from build123d import *

# Parameters (mm, degrees)
SKETCH1_R                      = 3.175
BOSS_EXTRUDE1_DEPTH            = 6.35
M2_CLEARANCE_HOLE1_D           = 2.4
M2_CLEARANCE_HOLE1_CSINK_D     = 2.45
M2_CLEARANCE_HOLE1_CSINK_ANGLE = 90


with BuildPart() as part:
    # Sketch1 → Boss-Extrude1 (new body)
    with BuildSketch(Plane.XY):
        Polygon((25.4, -6.35), (25.4, -7.9375), (-25.4, -7.9375), (-25.4, -6.35), (-19.05, -6.35), (-19.05, 6.35), (-25.4, 6.35), (-25.4, 7.9375), (25.4, 7.9375), (25.4, 6.35), (19.05, 6.35), (19.05, -6.35), align=None)
        Circle(SKETCH1_R, mode=Mode.SUBTRACT)
    extrude(amount=BOSS_EXTRUDE1_DEPTH)

    # Sketch4 → Tap Drill for #6-32 Tap1 (revolve, cut)
    with BuildSketch(Plane(origin=(19.05, 0, 3.175), x_dir=(0, 0, -1), z_dir=(0, 1, 0))):
        Polygon((0, 0), (0, 7.16269403), (1.35255, 6.35), (1.35255, 0), align=None)
    tap_drill_for_6_32_tap1 = revolve(axis=Axis((25.4, 0, 3.175), (-1, 0, 0)), mode=Mode.SUBTRACT)

    # M2 Clearance Hole1 (through all)
    with Locations(Plane(origin=(0, 0, 0), x_dir=(-1, 0, 0), z_dir=(0, 0, -1))):
        with Locations((-5.5, 0), (5.5, 0)):
            CounterSinkHole(M2_CLEARANCE_HOLE1_D / 2, M2_CLEARANCE_HOLE1_CSINK_D / 2, counter_sink_angle=M2_CLEARANCE_HOLE1_CSINK_ANGLE)

    # Mirror1: Tap Drill for #6-32 Tap1 across plane
    add(tap_drill_for_6_32_tap1.mirror(Plane.ZY), mode=Mode.SUBTRACT)


solid = part.part
Can you work these out from the model? Positions are in its coordinate system, mm. A direction names the side the tool comes from. Coordinates: 2 decimals unless noted, no trailing zeros. Order: outer loops, then holes, each group sorted by start corner. A loop starts at its lowest first (then second) coordinate and runs counter-clockwise, first axis right, second up. Notation, with made-up numbers: M -26,12 L -20,12 A15 ccw -20,34 Z; hole C 65.25,-5 d1. An arc over 180 degrees is marked long. Write item = value, one per line.
(1) Suppose I cut it at B-B on z = 1. State how many separate pieces and enclosed holes the cut face has, plus the area to 3 significant figures.
Results are:
separate_pieces = 1
enclosed_holes = 3
area = 604 mm2
(2) If we mould it in two halves opening along X, with no side actions, what happens to faces 1 (the face through (0, -7.938, 3)), 2 (the face through (19.05, 2, 3)), 3 (the face through (-6.7, 0.05, 3.23))? For each: pulls with the +X half, pulls with the -X half, needs draft (parallel to the pull), parting line crosses it, or undercut.
Results are:
face_1 = needs draft
face_2 = pulls with the +X half
face_3 = undercut
(3) For faces 4 (the face through (-19.05, -2, 3)), 5 (the face through (-12.028, 0.09, 2.958)), 6 (the face through (15.919, -0.059, 4.526)), 7 (the face through (22, 6.35, 3)), 8 (the face through (0.4, -3.4, 6.35)), which set-ups out of +Z, -Z, +X, -X, +Y, -Y let a thin tool reach every point of the face, with its end or its side?
Results are:
face_4 = +Z, -Z, -X
face_5 = -X
face_6 = +X
face_7 = +Z, -Z, +X
face_8 = +Z, +X, -X, +Y, -Y
(4) Suppose I cut it at C-C on y = -2. Please give me the cut outline in (x, z), plus the area to 3 significant figures.
Results are:
outline = M -19.05,0 L -2.47,0 L -2.47,6.35 L -19.05,6.35 Z; M 2.47,0 L 19.05,0 L 19.05,6.35 L 2.47,6.35 Z
area = 211 mm2
(5) For pin 1 Ø3 at (y, z) = (3, 1.5) entering from -X; pin 2 Ø3 at (y, z) = (0, 3.175) entering from +X; pin 3 Ø1.6 at (y, z) = (0, 3.175) entering from +X; pin 4 Ø5 at (x, y) = (-7.5, 1) entering from -Z, each with a flat end and sliding along its axis, tell me the tip position at first contact or that it passes through.
Results are:
pin_1 = -19.05
pin_2 = 19.05
pin_3 = 12.37
pin_4 = 0
(6) I need wall thicknesses on line 1 along Y through (x, z) = (0, 2.25) (1 decimal); line 2 along Z through (x, y) = (-15.5, 0); line 3 along Y through (x, z) = (-5.5, 2.5). Which ranges of each line are inside material? Lowest first, please. Write a range as [from, to].
Results are:
line_1 = [-7.9, -3.2], [3.2, 7.9]
line_2 = [0, 1.82], [4.53, 6.35]
line_3 = [-7.94, -1.2], [1.2, 7.94]
